Geometry: final body of the model. Coordinates: model frame, mm. A direction names the side the tool comes from. Round coordinates to 2 decimals unless told otherwise and drop trailing zeros. Loops run counter-clockwise (first coordinate to the right, second up) from the corner with the lowest first, then second, coordinate; pieces in that order, holes last. Notation, with made-up numbers: (23.25, 57) -> (47.25, 57) arc R17 ccw to (47.25, 63) -> close; hole circle Ø6 at (51, -33.5). An arc over 180 degrees is marked (long way). Answer in a Markdown table with one row per item.
```python
from build123d import *

# Parameters (mm, degrees)
SKETCH_1_R          = 10
SKETCH_1_R_2        = 1.65
EXTRUDE_1_DEPTH     = 3
SKETCH_2_R          = 3
EXTRUDE_2_DEPTH     = 80
SKETCH_3_W          = 2
SKETCH_3_H          = 7.743354912
CUT_EXTRUDE_1_DEPTH = 12
SKETCH_5_R          = 1
CUT_EXTRUDE_2_DEPTH = 5
SKETCH_6_R          = 4
EXTRUDE_3_DEPTH     = 45


with BuildPart() as part:
    # 草图1 → 凸台-拉伸1 (new body)
    with BuildSketch(Plane.XY):
        Circle(SKETCH_1_R)
        with Locations((0, 7)):
            Circle(SKETCH_1_R_2, mode=Mode.SUBTRACT)
        with Locations((7, 0)):
            Circle(SKETCH_1_R_2, mode=Mode.SUBTRACT)
        with Locations((0, -7)):
            Circle(SKETCH_1_R_2, mode=Mode.SUBTRACT)
        with Locations((-7, 0)):
            Circle(SKETCH_1_R_2, mode=Mode.SUBTRACT)
    extrude(amount=EXTRUDE_1_DEPTH)

    # 草图2 → 凸台-拉伸2 (add)
    with BuildSketch(Plane.XY.offset(3)):
        Circle(SKETCH_2_R)
    extrude(amount=EXTRUDE_2_DEPTH)

    # 草图3 → 切除-拉伸1 (cut)
    with BuildSketch(Plane.XY.offset(83)):
        Rectangle(SKETCH_3_W, SKETCH_3_H)
    extrude(amount=-CUT_EXTRUDE_1_DEPTH, mode=Mode.SUBTRACT)

    # 草图5 → 切除-拉伸2 (cut, symmetric)
    with BuildSketch(Plane(origin=(-1, 0, 0), x_dir=(0, 0, -1), z_dir=(1, 0, 0))):
        with Locations(Location((-80, 0, 0), (0, 0, 180))):
            Circle(SKETCH_5_R)
        with Locations(Location((-76, 0, 0), (0, 0, 180))):
            Circle(SKETCH_5_R)
    extrude(amount=CUT_EXTRUDE_2_DEPTH, both=True, mode=Mode.SUBTRACT)

    # 草图6 → 凸台-拉伸3 (add)
    with BuildSketch(Plane.XY.offset(3)):
        with Locations(Location((0, 0, 0), (0, 0, 180))):
            Circle(SKETCH_6_R)
    extrude(amount=EXTRUDE_3_DEPTH)


solid = part.part
```
Item 1: Cut plane B-B (x = 0). Output: boundary loops of the cut face in (y, z).
Answer:
| item | result |
|---|---|
| outline | (-10, 0) -> (-8.65, 0) -> (-8.65, 3) -> (-10, 3) -> close; (-5.35, 0) -> (5.35, 0) -> (5.35, 3) -> (4, 3) -> (4, 48) -> (3, 48) -> (3, 71) -> (-3, 71) -> (-3, 48) -> (-4, 48) -> (-4, 3) -> (-5.35, 3) -> close; (8.65, 0) -> (10, 0) -> (10, 3) -> (8.65, 3) -> close |
Item 2: Pin query (flat end, axial travel): pin 1 Ø6 at (y, z) = (-6, 21.5) entering from +X; pin 2 Ø3 at (x, z) = (-6, 53.5) entering from -Y; pin 3 Ø1.5 at (y, z) = (0.5, 19.5) entering from -X; pin 4 Ø5.5 at (x, y) = (0, 7) entering from +Z. Return the tip coordinate at first contact, or that it passes through.
Answer:
| item | result |
|---|---|
| pin 1 | stops at x = 2.65 |
| pin 2 | passes through |
| pin 3 | stops at x = -4 |
| pin 4 | stops at z = 3 |
Item 3: Cut plane A-A (z = 80). Output: boundary loops of the cut face in (x, y).
Answer:
| item | result |
|---|---|
| outline | (-2.83, -1) arc R3 ccw to (-1, -2.83) -> (-1, -1) -> close; (-2.83, 1) -> (-1, 1) -> (-1, 2.83) arc R3 ccw to start; (1, -2.83) arc R3 ccw to (2.83, -1) -> (1, -1) -> close; (1, 1) -> (2.83, 1) arc R3 ccw to (1, 2.83) -> close |
Item 4: Cut plane C-C (x = -7.5). Output: boundary loops of the cut face in (y, z).
Answer:
| item | result |
|---|---|
| outline | (-6.61, 0) -> (-1.57, 0) -> (-1.57, 3) -> (-6.61, 3) -> close; (1.57, 0) -> (6.61, 0) -> (6.61, 3) -> (1.57, 3) -> close |
Item 5: Cut plane D-D (z = 39.5). Output: boundary loops of the cut face in (x, y), then the cut area to 3 significant figures.
Answer:
| item | result |
|---|---|
| outline | circle Ø8 at (0, 0) |
| area | 50.3 mm² |
Item 6: Line query: probe 1 along Z at (x, y) = (-6.75, 3.75); probe 2 along Y at (x, z) = (1, 65); probe 3 along X at (y, z) = (-2, 74). Output: solid intervals per line, ascending. Write a range as [from, to].
Answer:
| item | result |
|---|---|
| probe 1 | z = [0, 3] |
| probe 2 | y = [-2.83, 2.83] |
| probe 3 | x = [-2.24, -1], [1, 2.24] |
Item 7: Reachability of faces 1 (the face through (0, 0, 71)), 2 (the face through (-1, -3, 48)), 3 (the face through (-2.17, -9.76, 1.48)) from +Z, -Z, +X, -X, +Y, -Y: full face, straight path, thin tool, end or side. Return the list, or none.
Answer:
| item | result |
|---|---|
| face 1 | +Z, +Y, -Y |
| face 2 | +Z |
| face 3 | +Z, -Z |
Item 8: Draft query along Y for faces 4 (the face through (-8.65, 0.07, 1.48)), 5 (the face through (-2, 0, 83)), 6 (the face through (5.35, 0.07, 1.48)), 7 (the face through (0.867, 3.905, 25.185)). Return one class per face: pulls with the +Y half, pulls with the -Y half, needs draft (parallel to the pull), parting line crosses it, or undercut.
Answer:
| item | result |
|---|---|
| face 4 | undercut |
| face 5 | needs draft |
| face 6 | undercut |
| face 7 | parting line crosses it |
